Autodesk Inventor part; units mm, degrees
ref_plane "YZ Plane" through (0, 0, 0) normal (1, 0, 0) x (0, 1, 0)
ref_plane "XZ Plane" through (0, 0, 0) normal (0, 1, 0) x (-1, 0, 0)
ref_plane "XY Plane" through (0, 0, 0) normal (0, 0, 1) x (1, 0, 0)
sketch "Skizze1" plane through (0, 0, 0) normal (0, 0, 1) x (1, 0, 0)
  line L0 (0, 0) -> (25, 0)
  line L1 (25, 0) -> (25, 30)
  line L2 (25, 30) -> (0, 30)
  line L3 (0, 30) -> (0, 0)
  dimension "d0" = 30
  dimension "d1" = 25
extrude "Extrusion1" add sketch "Skizze1" against normal blind 4
sketch "Skizze2" plane through (0, 0, 0) normal (0, 0, 1) x (1, 0, 0)
  circle A0 centre (12.5, 18) radius 8
  line L0 (25, 0) -> (25, 30)
  line L1 (0, 0) -> (25, 0)
  dimension "d4" = 16
  dimension "d5" = 12.5
  dimension "d6" = 18
extrude "Extrusion2" cut sketch "Skizze2" against normal blind 10
sketch "Skizze4" plane through (0, 0, 0) normal (0, 0, 1) x (1, 0, 0)
  line L0 (2.5, 13.3758) -> (22.5, 13.3758) construction
  line L1 (22.5, 13.3758) -> (22.5, 26.3758) construction
  line L2 (22.5, 26.3758) -> (2.5, 26.3758) construction
  line L3 (2.5, 26.3758) -> (2.5, 13.3758) construction
  line L4 (25, 0) -> (25, 30) construction
  circle A0 centre (2.5, 26.3758) radius 1.7
  circle A1 centre (22.5, 26.3758) radius 1.7
  circle A2 centre (22.5, 13.3758) radius 1.7
  circle A3 centre (2.5, 13.3758) radius 1.7
  point P0 (0, 0)
  point P1 (25, 3.0001)
  dimension "d12" = 20
  dimension "d13" = 13
  dimension "d14" = 2.5
  dimension "d15" = 3.4
  dimension "d16" = 3.4
  dimension "d17" = 3.4
  dimension "d18" = 3.4
extrude "Extrusion4" cut sketch "Skizze4" against normal blind 10
sketch "Skizze6" plane through (0, 0, 0) normal (0, 0, 1) x (1, 0, 0)
  line L0 (25, 0) -> (0, 0)
  line L1 (25, 0) -> (16, 0)
  line L2 (16, 0) -> (16, 6)
  line L3 (16, 6) -> (25, 6)
  line L4 (25, 6) -> (25, 0)
  line L5 (0, 0) -> (9, 0)
  line L6 (9, 0) -> (9, 6)
  line L7 (9, 6) -> (0, 6)
  line L8 (0, 6) -> (0, 0)
  line L9 (9, 6) -> (16, 6)
  line L10 (16, 6) -> (16, 0)
  line L11 (16, 0) -> (9, 0)
  line L12 (9, 0) -> (9, 6)
  dimension "d21" = 9
  dimension "d22" = 9
  dimension "d23" = 6
extrude "Extrusion5" cut sketch "Skizze6" against normal blind 10 contours L0 L6 L9 L2
sketch "Skizze7" plane through (0, 0, 0) normal (-1, 0, 0) x (0, 0, 1)
  circle A0 centre (-2, 2.5) radius 1.7
  line L0 (0, 30) -> (0, 0)
  line L1 (0, 0) -> (-4, 0)
  dimension "d26" = 3.4
  dimension "d27" = 2
  dimension "d28" = 2.5
extrude "Extrusion6" cut sketch "Skizze7" against normal blind 40
properties part number "kamera ot"
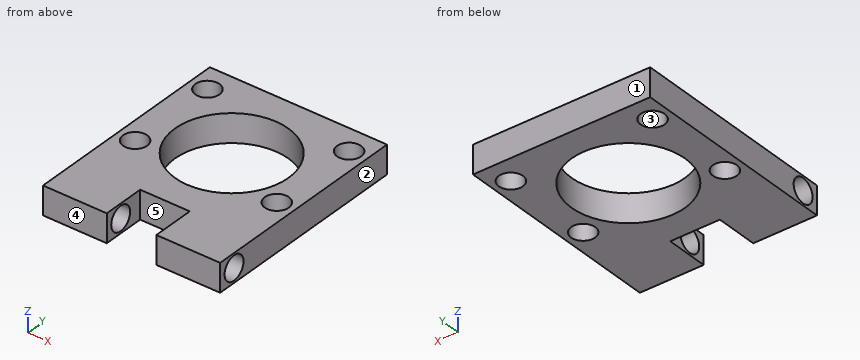
Input: part model. Units: mm. Frame: model coordinates. Face numbers are marked on the shaded views. A direction names the side the tool comes from. Give positions to 0.01 mm unless a question says otherwise; leave off trailing zeros. Order: outer loops, then holes, each group sorted by start corner. A loop starts at its lowest first (then second) coordinate and runs counter-clockwise, first axis right, second up.
1. Line query: probe 1 along Y at (x, z) = (22.5, -3.1); probe 2 along Y at (x, z) = (8.5, -1.8); probe 3 along Y at (x, z) = (19.25, -2). Output: solid intervals per line, ascending.
Computed:
probe 1: y = 0 to 1.2, 3.8 to 11.68, 15.08 to 24.68, 28.08 to 30
probe 2: y = 0 to 0.81, 4.19 to 11.07, 24.93 to 30
probe 3: y = 0 to 0.8, 4.2 to 13.71, 22.29 to 30
2. Cut plane D-D (x = 12.5). Return loops of the section in (y, z), and give its area (3 significant figures).
Computed:
outline: (6, -4) - (10, -4) - (10, 0) - (6, 0) - close; (26, -4) - (30, -4) - (30, 0) - (26, 0) - close
area: 32.0 mm2
3. Cut plane A-A (x = 2.5). Return loops of the section in (y, z), and give its area (3 significant figures).
Computed:
outline: (0, -4) - (11.68, -4) - (11.68, 0) - (0, 0) - close; (15.08, -4) - (24.68, -4) - (24.68, 0) - (15.08, 0) - close; (28.08, -4) - (30, -4) - (30, 0) - (28.08, 0) - close; hole circle Ø3.4 at (2.5, -2)
area: 83.7 mm2
4. Draft query along Y for the marked faces 1, 2 and 3. Return one class per face: released by +Y, released by -Y, zero draft, split by the parting line, or undercut.
Computed:
face 1: released by +Y
face 2: zero draft
face 3: undercut
5. Set-up query: the marked faces 4 and 5. Return all of +Z, -Z, +X, -X, +Y, -Y with unobstructed straight access to the full face (end or side cutting, diameter ignored); none if empty.
Computed:
face 4: +Z, -Z, +X, -X, -Y
face 5: +Z, -Z, -Y
6. Pin query (flat end, axial travel): pin 1 Ø2.5 at (x, y) = (2.5, 13.38) entering from -Z. Return the tip coordinate at first contact, or that it passes through.
Computed:
pin 1: passes through
7. Cut plane B-B (y = 2.5). Return loops of the section in (x, z), and give its area (3 significant figures).
Computed:
outline: (0, -4) - (9, -4) - (9, -3.7) - (0, -3.7) - close; (0, -0.3) - (9, -0.3) - (9, 0) - (0, 0) - close; (16, -4) - (25, -4) - (25, -3.7) - (16, -3.7) - close; (16, -0.3) - (25, -0.3) - (25, 0) - (16, 0) - close
area: 10.8 mm2
8. Cut plane C-C (z = -1.4). Return loops of the section in (x, y).
Computed:
outline: (0, 0) - (9, 0) - (9, 0.91) - (0, 0.91) - close; (0, 4.09) - (9, 4.09) - (9, 6) - (16, 6) - (16, 4.09) - (25, 4.09) - (25, 30) - (0, 30) - close; (16, 0) - (25, 0) - (25, 0.91) - (16, 0.91) - close; hole circle Ø3.4 at (2.5, 13.38); hole circle Ø3.4 at (2.5, 26.38); hole circle Ø16 at (12.5, 18); hole circle Ø3.4 at (22.5, 13.38); hole circle Ø3.4 at (22.5, 26.38)
